```python
from build123d import *

# Parameters (mm, degrees)
F0_R     = 19.05
F0_R_2   = 9.525
F1_DEPTH = 50.8
F3_W     = 38.1
F3_H     = 12.7
F4_DEPTH = 76.2
F6_R     = 12.7
F7_DEPTH = 6.35


with BuildPart() as f1:
    # F0 (on Top) → F1 (new body)
    with BuildSketch(Plane.XY):
        Circle(F0_R)
        Circle(F0_R_2, mode=Mode.SUBTRACT)
    extrude(amount=-F1_DEPTH)

    # F3 (on offset) → F4 (join)
    with BuildSketch(Plane.XZ.offset(38.1)):
        with Locations((1e-06, -25.4)):
            Rectangle(F3_W, F3_H)
    extrude(amount=-F4_DEPTH)

    # F6 (on offset) → F7 (cut)
    with BuildSketch(Plane.XY.offset(-6.35)):
        Circle(F6_R)
    extrude(amount=-F7_DEPTH, mode=Mode.SUBTRACT)


solid = f1.part
```
Could you check a few things on this model? Use its own coordinates, in mm. A direction names the side the tool comes from. Round coordinates to 2 decimals unless told otherwise and drop trailing zeros. Loops run counter-clockwise (first coordinate to the right, second up) from the corner with the lowest first, then second, coordinate; pieces in that order, holes last. Notation, with made-up numbers: (63, 65) - (74, 65) arc R16 cw to (74, 81) - close; hole circle Ø5 at (-16, -4). An arc over 180 degrees is marked (long way). Answer in a Markdown table with one row per item. Add a question column.
(1) If we section it at B-B (z = -17): Please give me the cut outline in (x, y) (3 decimals).
(2) I'm going to push flat-ended pins straight in: pin 1 (2 mm diameter, centred on x = 9, z = -37.5, fed in from +Y); pin 2 (17 mm diameter, centred on x = 0, y = 0, fed in from -Z); pin 3 (2 mm diameter, centred on x = -3, y = 1.5, fed in from +Z). Where does each tip first touch, or does it pass through?
(3) If we mould it in two halves opening along X, with no side actions, what happens to faces 5 (the face through (-19.05, 19, -25)), 6 (the face through (4, 9, 0)), 7 (the face through (-7.559, -5.796, -15.831))? For each: pulls with the +X half, pulls with the -X half, needs draft (parallel to the pull), parting line crosses it, or undercut.
(4) If we section it at D-D (y = 16): Please give me the cut outline in (x, z), plus the area to 3 significant figures.
(5) If we section it at C-C (y = 5): Please give me the cut outline in (x, z).
(6) I need wall thicknesses on line 1 along Y through (x, z) = (0, -14.5) (3 decimals); line 2 along Y through (x, z) = (0, -8.5); line 3 along Z through (x, y) = (-3, 33.5). Which ranges of each line are inside material? Lowest first, please.
(7) For faces 1 (the face through (5, 9, -12.7)), 2 (the face through (0, 0, -19.05)), 3 (the face through (19.05, -1, -25)), 4 (the face through (0, 0, -31.75)), which set-ups out of +Z, -Z, +X, -X, +Y, -Y let a thin tool reach every point of the face, with its end or its side?
(8) If we section it at A-A (x = 0): Please give me the cut outline in (y, z) (3 decimals), plus the area to 3 significant figures.
Model answer:
| question | item | result |
|---|---|---|
| 1 | outline | circle Ø38.1 at (0, 0); hole circle Ø19.05 at (0, 0) |
| 2 | pin 1 | stops at y = 17.29 |
| 2 | pin 2 | stops at z = -31.75 |
| 2 | pin 3 | stops at z = -19.05 |
| 3 | face 5 | pulls with the -X half |
| 3 | face 6 | needs draft |
| 3 | face 7 | undercut |
| 4 | outline | (-19.05, -31.75) - (-10.34, -31.75) - (-10.34, -50.8) - (10.34, -50.8) - (10.34, -31.75) - (19.05, -31.75) - (19.05, -19.05) - (10.34, -19.05) - (10.34, 0) - (-10.34, 0) - (-10.34, -19.05) - (-19.05, -19.05) - close |
| 4 | area | 1,270 mm² |
| 5 | outline | (-19.05, -31.75) - (-18.38, -31.75) - (-18.38, -50.8) - (-8.11, -50.8) - (-8.11, -31.75) - (8.11, -31.75) - (8.11, -50.8) - (18.38, -50.8) - (18.38, -31.75) - (19.05, -31.75) - (19.05, -19.05) - (18.38, -19.05) - (18.38, 0) - (8.11, 0) - (8.11, -6.35) - (11.67, -6.35) - (11.67, -12.7) - (8.11, -12.7) - (8.11, -19.05) - (-8.11, -19.05) - (-8.11, -12.7) - (-11.67, -12.7) - (-11.67, -6.35) - (-8.11, -6.35) - (-8.11, 0) - (-18.38, 0) - (-18.38, -19.05) - (-19.05, -19.05) - close |
| 6 | line 1 | y = -19.05 to -9.525, 9.525 to 19.05 |
| 6 | line 2 | y = -19.05 to -12.7, 12.7 to 19.05 |
| 6 | line 3 | z = -31.75 to -19.05 |
| 7 | face 1 | none |
| 7 | face 2 | +Z |
| 7 | face 3 | +Z, -Z, +X, +Y, -Y |
| 7 | face 4 | -Z |
| 8 | outline | (-38.1, -31.75) - (-19.05, -31.75) - (-19.05, -50.8) - (-9.525, -50.8) - (-9.525, -31.75) - (9.525, -31.75) - (9.525, -50.8) - (19.05, -50.8) - (19.05, -31.75) - (38.1, -31.75) - (38.1, -19.05) - (19.05, -19.05) - (19.05, 0) - (9.525, 0) - (9.525, -6.35) - (12.7, -6.35) - (12.7, -12.7) - (9.525, -12.7) - (9.525, -19.05) - (-9.525, -19.05) - (-9.525, -12.7) - (-12.7, -12.7) - (-12.7, -6.35) - (-9.525, -6.35) - (-9.525, 0) - (-19.05, 0) - (-19.05, -19.05) - (-38.1, -19.05) - close |
| 8 | area | 1,650 mm² |
